Here's the drawing with two shaded views (mm, measured from the low corner). I have some questions. A direction names the side the tool comes from. Give positions to 0.01 mm unless a question says otherwise; leave off trailing zeros. Write each loop counter-clockwise with the first axis right and the second up, starting at its lowest first coordinate (ties: lowest second). Pieces come first, ordered by that corner, then holes.
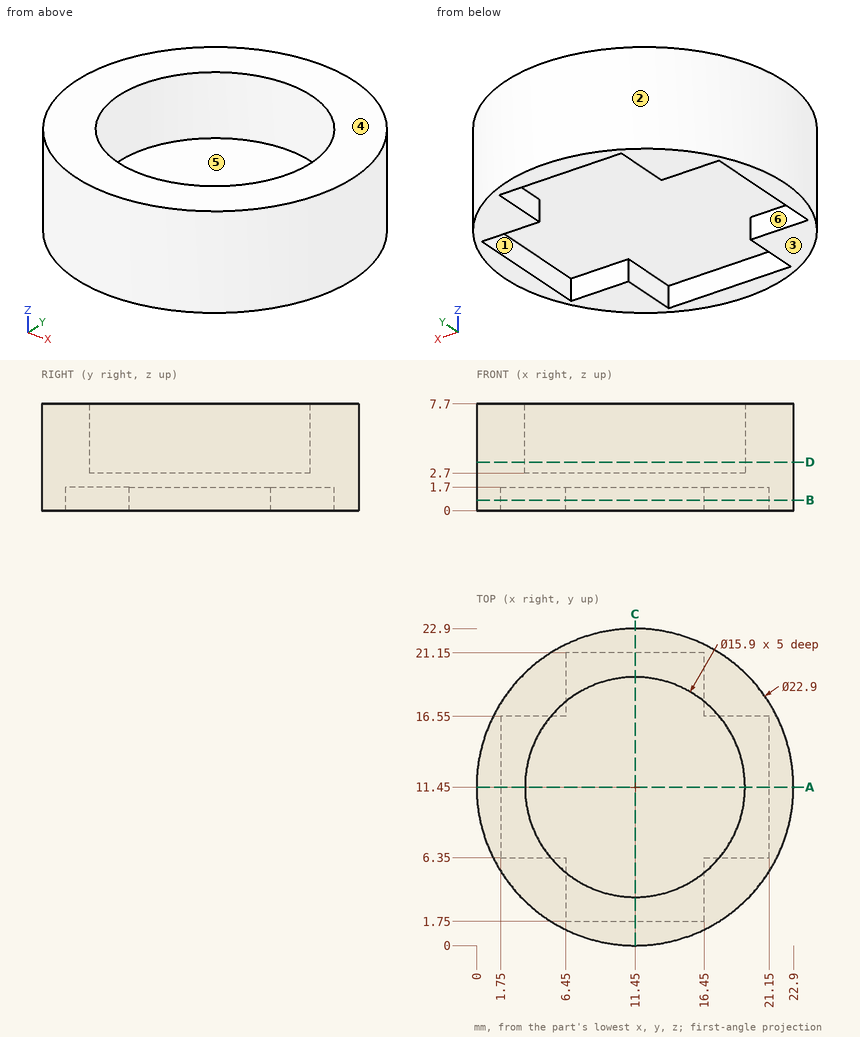
(1) Will these pins go through, and if not, where does the flat tip stop? P1, Ø0.8, axis at x = 19.5, z = 0.5, coming from the +Y side; P2, Ø0.5, axis at x = 12.5, z = 1, coming from the +Y side; P3, Ø1.4, axis at y = 3.5, z = 1, coming from the +X side; P4, Ø3, axis at x = 17.5, y = 7, coming from the -Z side.
Returned:
P1: stops at y = 19.97
P2: stops at y = 22.87
P3: stops at x = 20.31
P4: stops at z = 0
(2) Imagine slicing it at B-B, the plane z = 0.75. Write out the boundary of the cut face in (x, y).
Returned:
outline: circle Ø22.9 at (11.45, 11.45); hole (1.75, 6.35) - (6.45, 6.35) - (6.45, 1.75) - (16.45, 1.75) - (16.45, 6.35) - (21.15, 6.35) - (21.15, 16.55) - (16.45, 16.55) - (16.45, 21.15) - (6.45, 21.15) - (6.45, 16.55) - (1.75, 16.55) - close
(3) If I drill on L1, parallel to X at y = 11.75, z = 2.75; L2, parallel to Y at x = 11.45, z = 4.75; L3, parallel to Y at x = 14.25, z = 4.5, over which ranges is the centre line in solid material (lowest first)?
Returned:
L1: x = 0 to 3.51, 19.39 to 22.9
L2: y = 0 to 3.5, 19.4 to 22.9
L3: y = 0.35 to 4.01, 18.89 to 22.55
(4) For the marked faces 4, 5 and 6, which set-ups out of +Z, -Z, +X, -X, +Y, -Y let a thin tool reach every point of the face, with its end or its side?
Returned:
face 4: +Z, +X, -X, +Y, -Y
face 5: +Z
face 6: -Z
(5) Imagine slicing it at D-D, the plane z = 3.5. Write out the boundary of the cut face in (x, y), plus the area to 3 significant figures.
Returned:
outline: circle Ø22.9 at (11.45, 11.45); hole circle Ø15.9 at (11.45, 11.45)
area: 213 mm2
(6) If we mould it in two halves opening along Y, with no side actions, what happens to the marked faces 1, 2 and 3? For each: +Y half, -Y half, draft (parallel to the pull), parting line (faces both ways), or undercut.
Returned:
face 1: undercut
face 2: parting line
face 3: draft
(7) Imagine slicing it at A-A, the plane y = 11.45. Write out the boundary of the cut face in (x, z).
Returned:
outline: (0, 0) - (1.75, 0) - (1.75, 1.7) - (21.15, 1.7) - (21.15, 0) - (22.9, 0) - (22.9, 7.7) - (19.4, 7.7) - (19.4, 2.7) - (3.5, 2.7) - (3.5, 7.7) - (0, 7.7) - close
